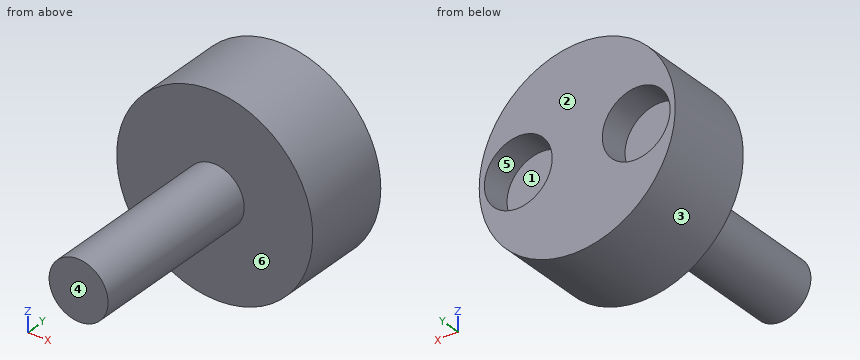
```python
from build123d import *

# Parameters (mm, degrees)
F0_R     = 6.65
F1_DEPTH = 6
F2_R     = 2
F3_DEPTH = 12
F4_R     = 2.3
F5_DEPTH = 2


with BuildPart() as f1:
    # F0 (on Front) → F1 (new body)
    with BuildSketch(Plane.XZ):
        Circle(F0_R)
    extrude(amount=F1_DEPTH)

    # F2 (on face) → F3 (join)
    with BuildSketch(Plane.XZ.offset(6)):
        Circle(F2_R)
    extrude(amount=F3_DEPTH)

    # F4 (on face) → F5 (cut)
    with BuildSketch(Plane(origin=(0, 0, 0), x_dir=(-1, 0, 0), z_dir=(0, 1, 0))):
        with Locations((-4, 0)):
            Circle(F4_R)
        with Locations((4, 0)):
            Circle(F4_R)
    extrude(amount=-F5_DEPTH, mode=Mode.SUBTRACT)


solid = f1.part
```
Work out the finished part from the listing and answer in its coordinate system (mm). Face numbers are marked on the shaded views. A direction names the side the tool comes from. Coordinates: 2 decimals unless noted, no trailing zeros. Write each loop counter-clockwise with the first axis right and the second up, starting at its lowest first coordinate (ties: lowest second). Pieces come first, ordered by that corner, then holes.
Q1. Each of these flat-tipped pins is pushed along its axis until it touches: pin 1 Ø1.4 at (x, z) = (4, 0.5) entering from +Y; pin 2 Ø2 at (y, z) = (-8.5, -1.5) entering from -X; pin 3 Ø6 at (y, z) = (-9.5, -3) entering from -X. Where does it stop, or does it pass through?
Q2. Determine the mould class of the marked faces 1, 2 and 3 for opening direction Z: released by +Z, released by -Z, zero draft, split by the parting line, or undercut.
Q3. A cutting plane is placed at D-D, the plane x = -4. Give the vertices of the cut face in (y, z), then the cut area to 3 significant figures.
Q4. Find the intervals of material crossed by line 1 (Y direction, x = 4, z = -1); line 2 (Y direction, x = -1.75, z = 5.75); line 3 (Z direction, x = -4, y = -0.6), in increasing order.
Q5. Which of the six approach directions +Z, -Z, +X, -X, +Y, -Y give full straight-line access (tool end or side, diameter ignored) to the marked faces 4, 5 and 6?
Q6. A cutting plane is placed at B-B, the plane z = 0. Give the vertices of the cut face in (x, y).
Q7. A cutting plane is placed at A-A, the plane x = 0. Give the vertices of the cut face in (y, z).
Q8. A cutting plane is placed at C-C, the plane y = -3.5. Give the vertices of the cut face in (x, z).
Findings below:
1. pin 1: stops at y = -2
1. pin 2: stops at x = -1.94
1. pin 3: stops at x = -2
2. face 1: undercut
2. face 2: zero draft
2. face 3: split by the parting line
3. outline: (-6, -5.31) - (0, -5.31) - (0, -2.3) - (-2, -2.3) - (-2, 2.3) - (0, 2.3) - (0, 5.31) - (-6, 5.31) - close
3. area: 54.5 mm2
4. line 1: y = -6 to -2
4. line 2: y = -6 to 0
4. line 3: z = -5.31 to -2.3, 2.3 to 5.31
5. face 4: +Z, -Z, +X, -X, -Y
5. face 5: +Y
5. face 6: -Y
6. outline: (-6.65, -6) - (-2, -6) - (-2, -18) - (2, -18) - (2, -6) - (6.65, -6) - (6.65, 0) - (6.3, 0) - (6.3, -2) - (1.7, -2) - (1.7, 0) - (-1.7, 0) - (-1.7, -2) - (-6.3, -2) - (-6.3, 0) - (-6.65, 0) - close
7. outline: (-18, -2) - (-6, -2) - (-6, -6.65) - (0, -6.65) - (0, 6.65) - (-6, 6.65) - (-6, 2) - (-18, 2) - close
8. outline: circle Ø13.3 at (0, 0)
